The listing builds one solid part. Answer for the finished solid, in the listing's coordinates (mm). Face numbers are marked on the shaded views. Coordinates: 2 decimals unless noted, no trailing zeros. Order: outer loops, then holes, each group sorted by start corner. A loop starts at its lowest first (then second) coordinate and runs counter-clockwise, first axis right, second up.
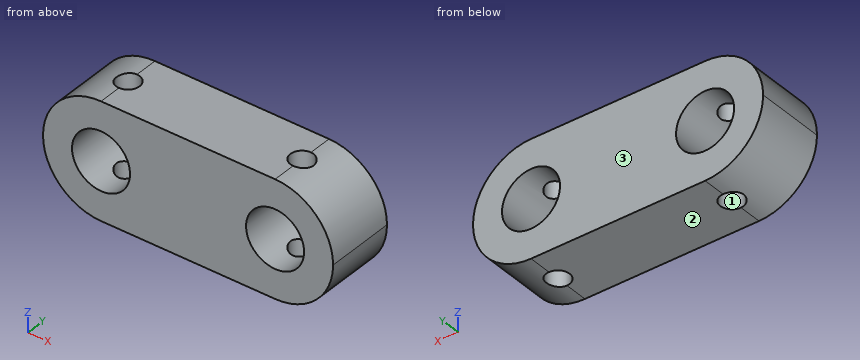
from build123d import *

# Parameters (mm, degrees)
SKETCH_1_W          = 75
SKETCH_1_H          = 18
EXTRUDE_1_DEPTH     = 30
SKETCH_9_R          = 7.5
CUT_EXTRUDE_6_DEPTH = 100
FILLET_1_R          = 15
SKETCH_10_R         = 7.5
CUT_EXTRUDE_7_DEPTH = 50
SKETCH_11_R         = 3
CUT_EXTRUDE_8_DEPTH = 60


with BuildPart() as part:
    # 草图1 → 拉伸1 (new body)
    with BuildSketch(Plane.XY):
        with Locations((37.5, -9)):
            Rectangle(SKETCH_1_W, SKETCH_1_H)
    extrude(amount=EXTRUDE_1_DEPTH)

    # 草图9 → 切除-拉伸6 (cut)
    with BuildSketch(Plane(origin=(0, 0, 0), x_dir=(1, 0, 0), z_dir=(0, 1, 0))):
        with Locations(Location((15, -15, 0), (0, 0, 270))):
            Circle(SKETCH_9_R)
    extrude(amount=-CUT_EXTRUDE_6_DEPTH, mode=Mode.SUBTRACT)

    # 圆角1
    fillet_1_edges = [part.edges().sort_by_distance(p)[0] for p in [
        (75, -9, 0),
        (75, -9, 30),
        (0, -9, 0),
        (0, -9, 30),
    ]]
    fillet(fillet_1_edges, radius=FILLET_1_R - 0.0001)  # a hair under: the kernel refuses the full size

    # 草图10 → 切除-拉伸7 (cut)
    with BuildSketch(Plane.XZ.offset(18)):
        with Locations(Location((60, 15, 0), (0, 0, 270))):
            Circle(SKETCH_10_R)
    extrude(amount=-CUT_EXTRUDE_7_DEPTH, mode=Mode.SUBTRACT)

    # 草图11 → 切除-拉伸8 (cut)
    with BuildSketch(Plane(origin=(0, 0, 0), x_dir=(-1, 0, 0), z_dir=(0, 0, -1))):
        with Locations((-60, -9)):
            Circle(SKETCH_11_R)
        with Locations((-15, -9)):
            Circle(SKETCH_11_R)
    extrude(amount=-CUT_EXTRUDE_8_DEPTH, mode=Mode.SUBTRACT)


solid = part.part
(1) Find section B-B on x = 64. Determine the outline of the cut face in (y, z).
(2) Given pin 1 Ø9.5 at (x, y) = (15, -9) entering from +Z; pin 2 Ø4 at (x, y) = (11, -3.5) entering from -Z, each flat-ended and moving along its own axis, determine where each tip first touches the part or whether it passes through.
(3) Find section C-C on z = 16.5. Determine the outline of the cut face in (x, y).
(4) The mould has two halves that part along Y. Classify the marked faces 1, 2 and 3: pulls with the +Y half, pulls with the -Y half, needs draft (parallel to the pull), parting line crosses it, or undercut.
(5) Find the intervals of material crossed by probe 1 along X at (y, z) = (-9.5, 15); probe 2 along X at (y, z) = (-3, 21); probe 3 along Y at (x, z) = (15, 4), in increasing order.
(6) Find section A-A on y = -14.75. Count the separate pieces of the cut face and the enclosed holes in it, then the cut area to 3 significant figures.
Resolved:
1. outline: (-18, 0.54) - (0, 0.54) - (0, 8.66) - (-18, 8.66) - close; (-18, 21.34) - (0, 21.34) - (0, 29.46) - (-18, 29.46) - close
2. pin 1: stops at z = 30
2. pin 2: stops at z = 0.13
3. outline: (0.08, -18) - (7.65, -18) - (7.65, 0) - (0.08, 0) - close; (22.35, -18) - (52.65, -18) - (52.65, 0) - (22.35, 0) - close; (67.35, -18) - (74.92, -18) - (74.92, 0) - (67.35, 0) - close
4. face 1: undercut
4. face 2: needs draft
4. face 3: pulls with the +Y half
5. probe 1: x = 0 to 7.5, 22.5 to 52.5, 67.5 to 75
5. probe 2: x = 1.25 to 10.5, 19.5 to 55.5, 64.5 to 73.75
5. probe 3: y = -18 to -12, -6 to 0
6. separate pieces: 1
6. enclosed holes: 2
6. area: 1,700 mm2
